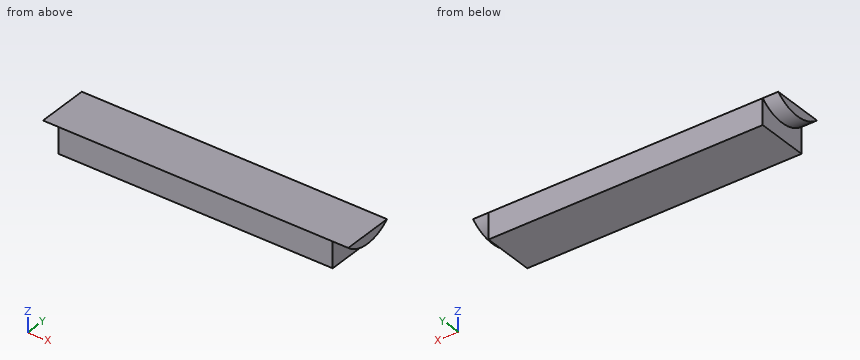
from build123d import *

# Parameters (mm, degrees)
SKETCH_1_W      = 53
SKETCH_1_H      = 10
EXTRUDE_1_DEPTH = 5
EXTRUDE_2_DEPTH = 3
EXTRUDE_START   = 3
EXTRUDE_3_DEPTH = 3


with BuildPart() as part:
    # 草图1 → 凸台-拉伸1 (new body)
    with BuildSketch(Plane.XY):
        Rectangle(SKETCH_1_W, SKETCH_1_H)
    extrude(amount=EXTRUDE_1_DEPTH)

    # 草图2 → 凸台-拉伸2 (add)
    with BuildSketch(Plane(origin=(26.5, 0, 0), x_dir=(0, 0, -1), z_dir=(1, 0, 0))):
        with BuildLine():
            Line((-5, 5), (-5, -5))
            ThreePointArc((-5, -5), (-3.090169944, 0), (-5, 5))
        make_face()
    extrude(amount=EXTRUDE_2_DEPTH)

    # 草图3 → 凸台-拉伸3 (add)
    with BuildSketch(Plane.ZY.offset(26.5).offset(EXTRUDE_START)):
        with BuildLine():
            Line((5, -5), (5, 5))
            ThreePointArc((5, 5), (3.090169944, 0), (5, -5))
        make_face()
    extrude(amount=-EXTRUDE_3_DEPTH)


solid = part.part
Here's how the part is built. I have some questions about the finished solid (model axes, mm). Coordinates: 2 decimals unless noted, no trailing zeros. Write each loop counter-clockwise with the first axis right and the second up, starting at its lowest first coordinate (ties: lowest second). Pieces come first, ordered by that corner, then holes.
1) If we section it at A-A (y = -2): List the corners of the cut face in (x, z) for me, plus the area to 3 significant figures.
Filled in:
outline: (-29.5, 3.36) - (-26.5, 3.36) - (-26.5, 0) - (26.5, 0) - (26.5, 3.36) - (29.5, 3.36) - (29.5, 5) - (-29.5, 5) - close
area: 275 mm2
2) If we section it at C-C (z = 1.6): List the corners of the cut face in (x, y) for me, plus the area to 3 significant figures.
Filled in:
outline: (-26.5, -5) - (26.5, -5) - (26.5, 5) - (-26.5, 5) - close
area: 530 mm2
3) If I drill on line 1 (X direction, y = 0.75, z = 0.4); line 2 (Z direction, x = -27, y = 1.25), over which ranges is the centre line in solid material (lowest first)?
Filled in:
line 1: x = -26.5 to 26.5
line 2: z = 3.2 to 5
4) If we section it at B-B (z = 4.1): List the corners of the cut face in (x, y) for me.
Filled in:
outline: (-29.5, -3.76) - (-26.5, -3.76) - (-26.5, -5) - (26.5, -5) - (26.5, -3.76) - (29.5, -3.76) - (29.5, 3.76) - (26.5, 3.76) - (26.5, 5) - (-26.5, 5) - (-26.5, 3.76) - (-29.5, 3.76) - close
